Can you work these out from the model? Positions are in its coordinate system, mm. Give positions to 0.01 mm unless a question says otherwise; leave off trailing zeros. Order: outer loops, then holes, each group sorted by start corner. A loop starts at its lowest first (then second) coordinate and runs counter-clockwise, first axis right, second up. Notation, with made-up numbers: M -24,57.25 L -6,57.25 A26 ccw -6,88.25 Z; hole C -17,64.25 d1. An arc over 180 degrees is marked long. Answer as a JSON object with one key per item and string values.
```python
from build123d import *

# Parameters (mm, degrees)
BOSS_EXTRUDE1_DEPTH = 4
SKETCH2_R           = 4.5
SKETCH2_R_2         = 6
CUT_EXTRUDE1_DEPTH  = 10
SKETCH3_R           = 1.6
CUT_EXTRUDE2_DEPTH  = 10
SKETCH4_R           = 35
CUT_EXTRUDE3_DEPTH  = 10
SKETCH5_R           = 1.5
CUT_EXTRUDE4_DEPTH  = 10


with BuildPart() as part:
    # Sketch1 → Boss-Extrude1 (new body)
    with BuildSketch(Plane(origin=(0, 0, 0), x_dir=(1, 0, 0), z_dir=(0, 1, 0))):
        with BuildLine():
            ThreePointArc((14.123893805, 43.357532492), (-45.6, 0), (14.123893805, -43.357532492))
            Line((14.123893805, -43.357532492), (27.105327803, -39.128777194))
            ThreePointArc((27.105327803, -39.128777194), (32.307019566, -34.957352399), (36.874788135, -30.1))
            Line((36.874788135, -30.1), (54.821870135, -30.1))
            Line((54.821870135, -30.1), (65.203539823, -26.718128575))
            ThreePointArc((65.203539823, -26.718128575), (84.6, 0), (65.203539823, 26.718128575))
            Line((65.203539823, 26.718128575), (14.123893805, 43.357532492))
        make_face()
    extrude(amount=BOSS_EXTRUDE1_DEPTH)

    # Sketch2 → Cut-Extrude1 (cut)
    with BuildSketch(Plane(origin=(0, 4, 0), x_dir=(1, 0, 0), z_dir=(0, 1, 0))):
        with Locations(Location((0, 0, 0), (0, 0, 270))):
            Circle(SKETCH2_R)
        with Locations(Location((56.5, 0, 0), (0, 0, 270))):
            Circle(SKETCH2_R_2)
    extrude(amount=-CUT_EXTRUDE1_DEPTH, mode=Mode.SUBTRACT)

    # Sketch3 → Cut-Extrude2 (cut)
    with BuildSketch(Plane(origin=(0, 4, 0), x_dir=(1, 0, 0), z_dir=(0, 1, 0))):
        with Locations(Location((78.583647797, 12.75, 0), (0, 0, 270))):
            Circle(SKETCH3_R)
        with Locations(Location((-21.5, 37.239092363, 0), (0, 0, 270))):
            Circle(SKETCH3_R)
        with Locations(Location((-21.5, -37.239092363, 0), (0, 0, 270))):
            Circle(SKETCH3_R)
    extrude(amount=-CUT_EXTRUDE2_DEPTH, mode=Mode.SUBTRACT)

    # Sketch4 → Cut-Extrude3 (cut)
    with BuildSketch(Plane(origin=(0, 4, 0), x_dir=(1, 0, 0), z_dir=(0, 1, 0))):
        with Locations(Location((0, 0, 0), (0, 0, 270))):
            Circle(SKETCH4_R)
    extrude(amount=-CUT_EXTRUDE3_DEPTH, mode=Mode.SUBTRACT)

    # Sketch5 → Cut-Extrude4 (cut)
    with BuildSketch(Plane(origin=(0, 4, 0), x_dir=(1, 0, 0), z_dir=(0, 1, 0))):
        with Locations(Location((48.781600067, -10.329892746, 0), (0, 0, 270))):
            Circle(SKETCH5_R)
        with Locations(Location((66.758977017, -7.491950177, 0), (0, 0, 270))):
            Circle(SKETCH5_R)
        with Locations(Location((61.613256974, 25.104392643, 0), (0, 0, 270))):
            Circle(SKETCH5_R)
        with Locations(Location((43.635880025, 22.266450075, 0), (0, 0, 270))):
            Circle(SKETCH5_R)
    extrude(amount=-CUT_EXTRUDE4_DEPTH, mode=Mode.SUBTRACT)


solid = part.part
```
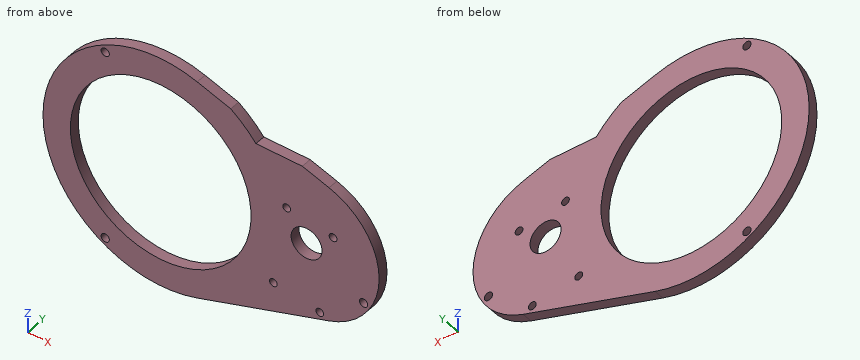
1) I want a section at C-C on x = -21.5. Write out the boundary of the cut face in (y, z).
Results found:
{"outline": "M 0,-40.21 L 4,-40.21 L 4,-38.84 L 0,-38.84 Z; M 0,-35.64 L 4,-35.64 L 4,-27.62 L 0,-27.62 Z; M 0,27.62 L 4,27.62 L 4,35.64 L 0,35.64 Z; M 0,38.84 L 4,38.84 L 4,40.21 L 0,40.21 Z"}
2) I want a section at A-A on x = 0. Write out the boundary of the cut face in (y, z).
Results found:
{"outline": "M 0,-45.6 L 4,-45.6 L 4,-35 L 0,-35 Z; M 0,35 L 4,35 L 4,45.6 L 0,45.6 Z"}
3) I need wall thicknesses on L1, parallel to X at y = 1.65, z = -5; L2, parallel to X at y = 1.3, z = -12.75; L3, parallel to Z at x = -28.5, y = 2.1. Which ranges of each line are inside material? Lowest first, please.
Results found:
{"L1": "x = -45.33 to -34.64, 34.64 to 53.18, 59.82 to 84.15", "L2": "x = -43.78 to -32.6, 32.6 to 76.98, 80.18 to 81.54", "L3": "z = -35.6 to -20.32, 20.32 to 35.6"}
4) I want a section at D-D on y = 2.6. Count the separate pieces of the cut face and the enclosed holes in it, and give its area (3 significant figures).
Results found:
{"separate pieces": "1", "enclosed holes": "9", "area": "4,780 mm²"}
5) I'm going to push flat-ended pins straight in: pin 1 Ø2.5 at (x, z) = (61.61, -25.1) entering from +Y; pin 2 Ø5 at (x, z) = (52, 19.5) entering from -Y; pin 3 Ø1.5 at (x, y) = (42.5, 2) entering from +Z. Where does each tip first touch, or does it pass through?
Results found:
{"pin 1": "passes through", "pin 2": "stops at y = 0", "pin 3": "stops at z = 30.1"}
6) I want a section at B-B on z = 0. Write out the boundary of the cut face in (x, y).
Results found:
{"outline": "M -45.6,0 L -35,0 L -35,4 L -45.6,4 Z; M 35,0 L 50.5,0 L 50.5,4 L 35,4 Z; M 62.5,0 L 84.6,0 L 84.6,4 L 62.5,4 Z"}
